Design review of the part built by this model. Coordinates are the model's own, in mm. A direction names the side the tool comes from. Coordinates: 2 decimals unless noted, no trailing zeros. Order: outer loops, then holes, each group sorted by start corner. A loop starts at its lowest first (then second) coordinate and runs counter-clockwise, first axis right, second up. Notation, with made-up numbers: M -4.75,1 L 29.25,1 A25 ccw 29.25,23 Z; hole C 65.5,59 d9. An arc over 180 degrees is marked long. Answer as a JSON object with one key per item and string values.
from build123d import *

# Parameters (mm, degrees)
SKETCH2_R          = 2.5
SKETCH2_W          = 30
SKETCH2_H          = 110
CUT_EXTRUDE1_DEPTH = 507.87769728
SKETCH3_R          = 1.5
CUT_EXTRUDE2_DEPTH = 476.279917621
CUT_EXTRUDE3_REACH = 501.074
SKETCH4_R          = 2.5


with BuildPart() as part:
    # Sketch1 → Revolve1 (revolve)
    with BuildSketch(Plane.XY, mode=Mode.PRIVATE) as revolve1_sk:
        Polygon((20, 0), (45, 0), (45, 5), (25, 5), (25, 500), (17.5, 500), (17.5, 496), (12.5, 496), (12.5, 471), (6, 471), (6, 464), (20, 464), align=None)
    revolve(revolve1_sk.sketch.rotate(Axis((0, 0, 0), (0, 1, 0)), 90), axis=Axis((0, 0, 0), (0, 1, 0)))

    # Sketch2 → Cut-Extrude1 (cut, through all)
    with BuildSketch(Plane.ZY.offset(25)):
        with Locations((0, 299)):
            Circle(SKETCH2_R)
        with Locations((15, 409)):
            Rectangle(SKETCH2_W, SKETCH2_H)
    extrude(amount=-CUT_EXTRUDE1_DEPTH, mode=Mode.SUBTRACT)

    # Sketch3 → Cut-Extrude2 (cut, through all)
    with BuildSketch(Plane(origin=(0, 471, 0), x_dir=(1, 0, 0), z_dir=(0, 1, 0))):
        with Locations(Location((-8.090824797, 5.99528599, 0), (0, 0, 270))):
            Circle(SKETCH3_R)
        with Locations(Location((7.409175203, 6.819752401, 0), (0, 0, 270))):
            Circle(SKETCH3_R)
    extrude(amount=-CUT_EXTRUDE2_DEPTH, mode=Mode.SUBTRACT)

    # Sketch4 → Cut-Extrude3 (cut, up to next)
    with BuildSketch(Plane(origin=(0, 5, 0), x_dir=(1, 0, 0), z_dir=(0, 1, 0)), mode=Mode.PRIVATE) as cut_extrude3_sk1:
        with Locations(Location((0, 35, 0), (0, 0, 270))):
            Circle(SKETCH4_R)
    cut_extrude3_tool1 = extrude(cut_extrude3_sk1.sketch, amount=-CUT_EXTRUDE3_REACH, mode=Mode.PRIVATE) & part.part
    # Sketch4 → Cut-Extrude3 (cut, up to next)
    with BuildSketch(Plane(origin=(0, 5, 0), x_dir=(1, 0, 0), z_dir=(0, 1, 0)), mode=Mode.PRIVATE) as cut_extrude3_sk2:
        with Locations(Location((35, 0, 0), (0, 0, 270))):
            Circle(SKETCH4_R)
    cut_extrude3_tool2 = extrude(cut_extrude3_sk2.sketch, amount=-CUT_EXTRUDE3_REACH, mode=Mode.PRIVATE) & part.part
    # Sketch4 → Cut-Extrude3 (cut, up to next)
    with BuildSketch(Plane(origin=(0, 5, 0), x_dir=(1, 0, 0), z_dir=(0, 1, 0)), mode=Mode.PRIVATE) as cut_extrude3_sk3:
        with Locations(Location((0, -35, 0), (0, 0, 270))):
            Circle(SKETCH4_R)
    cut_extrude3_tool3 = extrude(cut_extrude3_sk3.sketch, amount=-CUT_EXTRUDE3_REACH, mode=Mode.PRIVATE) & part.part
    # Sketch4 → Cut-Extrude3 (cut, up to next)
    with BuildSketch(Plane(origin=(0, 5, 0), x_dir=(1, 0, 0), z_dir=(0, 1, 0)), mode=Mode.PRIVATE) as cut_extrude3_sk4:
        with Locations(Location((-35, 0, 0), (0, 0, 270))):
            Circle(SKETCH4_R)
    cut_extrude3_tool4 = extrude(cut_extrude3_sk4.sketch, amount=-CUT_EXTRUDE3_REACH, mode=Mode.PRIVATE) & part.part
    add(cut_extrude3_tool1.solids().sort_by_distance((0, 5, -35))[0], mode=Mode.SUBTRACT)
    add(cut_extrude3_tool2.solids().sort_by_distance((35, 5, 0))[0], mode=Mode.SUBTRACT)
    add(cut_extrude3_tool3.solids().sort_by_distance((0, 5, 35))[0], mode=Mode.SUBTRACT)
    add(cut_extrude3_tool4.solids().sort_by_distance((-35, 5, 0))[0], mode=Mode.SUBTRACT)


solid = part.part
1) Add section A-A (y = 64). State the section outline as (x, z) points, and give its area (3 significant figures).
Taken from the geometry:
{"outline": "C 0,0 d50; hole C 0,0 d40", "area": "707 mm2"}
2) Mouldability with a two-part tool opening along X and no side actions: class faces 6 (the flat face through (5, 500, 17)), 7 (the cylindrical face through (-1.802, 467.451, -5.723)), 8 (the cylindrical face through (39.923, 2.535, -20.765)) as released by +X, released by -X, zero draft, split by the parting line, or undercut.
Taken from the geometry:
{"face 6": "zero draft", "face 7": "undercut", "face 8": "split by the parting line"}
3) To check wall thickness, follow L1, parallel to X at y = 2, z = 0; L2, parallel to X at y = 80.5, z = 2; L3, parallel to X at y = 267, z = 0. State the ranges of each line that lie inside material, in increasing order.
Taken from the geometry:
{"L1": "x = -45 to -37.5, -32.5 to -20, 20 to 32.5, 37.5 to 45", "L2": "x = -24.92 to -19.9, 19.9 to 24.92", "L3": "x = -25 to -20, 20 to 25"}
4) Insertion check: pin 1 Ø6.5 at (x, z) = (0, 35) entering from -Y; pin 2 Ø12 at (x, y) = (-17.5, 174) entering from +Z; pin 3 Ø2 at (y, z) = (333, 12) entering from -X; pin 4 Ø20 at (x, z) = (0, 0) entering from -Y. Each pin has a flat end and moves straight along its axis. Give the tip position at first contact, or say it passes through.
Taken from the geometry:
{"pin 1": "stops at y = 0", "pin 2": "stops at z = 22.2", "pin 3": "stops at x = -22.45", "pin 4": "stops at y = 464"}
5) Tool access review of faces 1 (the flat face through (0, 464, 7)), 2 (the cylindrical face through (17.084, 497.972, 3.794)), 3 (the flat face through (-4, 354, 20)), 4 (the cylindrical face through (-6.007, 228.752, -19.076)), 5 (the flat face through (19, 0, 9)): name each direction out of +Z, -Z, +X, -X, +Y, -Y from which nothing blocks a thin tool from reaching the whole face with its end or side.
Taken from the geometry:
{"face 1": "+Z", "face 2": "+Y", "face 3": "+Z, +X, -X", "face 4": "-Y", "face 5": "+Z, -Z, +X, -X, -Y"}
